Source: three-view drawing plus pictorial views. Frame: mm from the lowest corner of the part. A direction names the side the tool comes from. Give positions to 0.01 mm unless a question says otherwise; leave off trailing zeros. Loops run counter-clockwise (first coordinate to the right, second up) from the corner with the lowest first, then second, coordinate; pieces in that order, holes last. Notation, with made-up numbers: M -5.75,51 L 46.25,51 A21 cw 46.25,66 Z; hole C 19,-10.5 d3. An arc over 180 degrees is marked long. Write item = value, one per line.
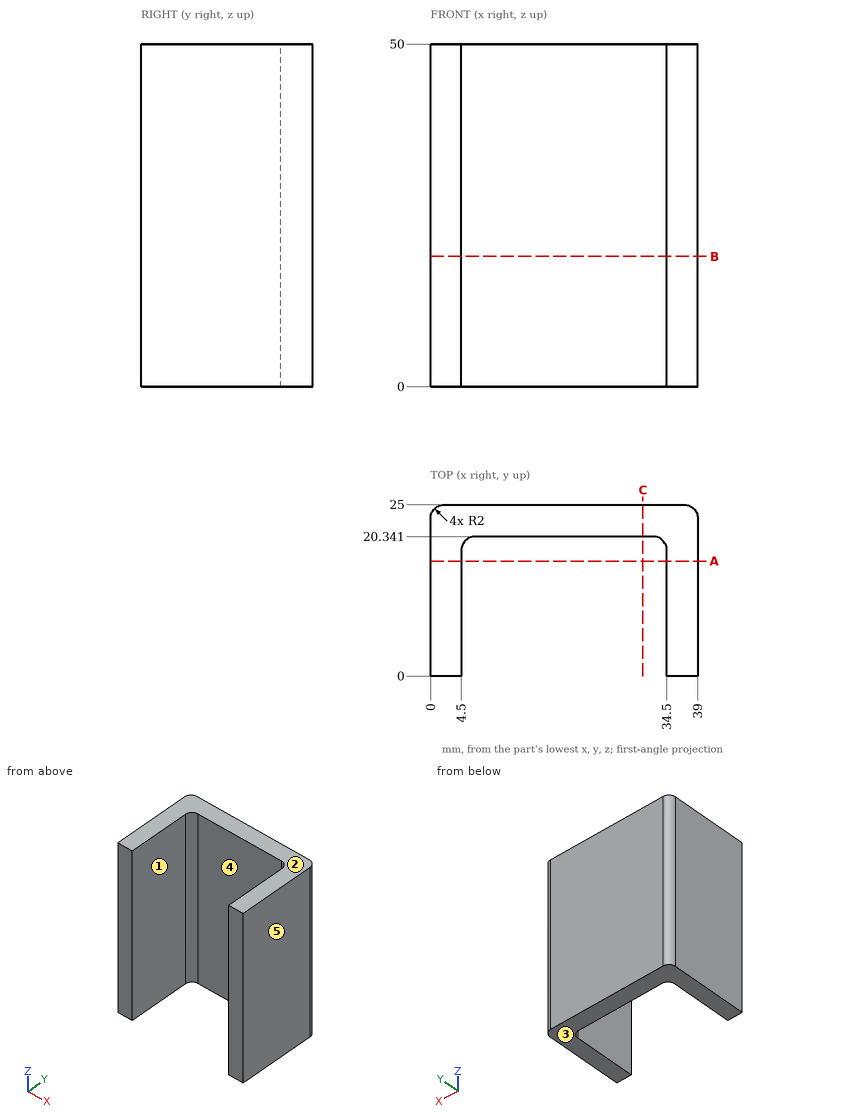
1. Cut plane B-B, the plane z = 19. Return the cut outline in (x, y).
Derived:
outline = M 0,0 L 4.5,0 L 4.5,18.34 A2 cw 6.5,20.34 L 32.5,20.34 A2 cw 34.5,18.34 L 34.5,0 L 39,0 L 39,23 A2 ccw 37,25 L 2,25 A2 ccw 0,23 Z
2. First-contact query: pin 1 Ø13 at (x, z) = (20.5, 24.5) entering from -Y. Flat tip, straight axial feed; report the tip coordinate or a pass-through.
Derived:
pin_1 = 20.34
3. Cut plane C-C, the plane x = 31. Return the cut outline in (y, z).
Derived:
outline = M 20.34,0 L 25,0 L 25,50 L 20.34,50 Z
4. Pull-direction query (X, two-part tool) for the marked faces 3, 4 and 5; classes: +X half, -X half, draft (parallel to the pull), parting line (faces both ways), or undercut.
Derived:
face_3 = draft
face_4 = undercut
face_5 = +X half
5. Material intervals for probe 1 along X at (y, z) = (9, 21); probe 2 along Y at (x, z) = (12.5, 28); probe 3 along X at (y, z) = (19.25, 25), sorted ascending. Write a range as from..to.
Derived:
probe_1 = 0..4.5, 34.5..39
probe_2 = 20.34..25
probe_3 = 0..4.72, 34.28..39
6. Reachability of the marked faces 1 and 2 from +Z, -Z, +X, -X, +Y, -Y: full face, straight path, thin tool, end or side. Return the list, or none.
Derived:
face_1 = +Z, -Z, -Y
face_2 = +Z, +X, -X, +Y, -Y
7. Cut plane A-A, the plane y = 16.75. Return the cut outline in (x, z), then the cut area to 3 significant figures.
Derived:
outline = M 0,0 L 4.5,0 L 4.5,50 L 0,50 Z; M 34.5,0 L 39,0 L 39,50 L 34.5,50 Z
area = 450 mm²
